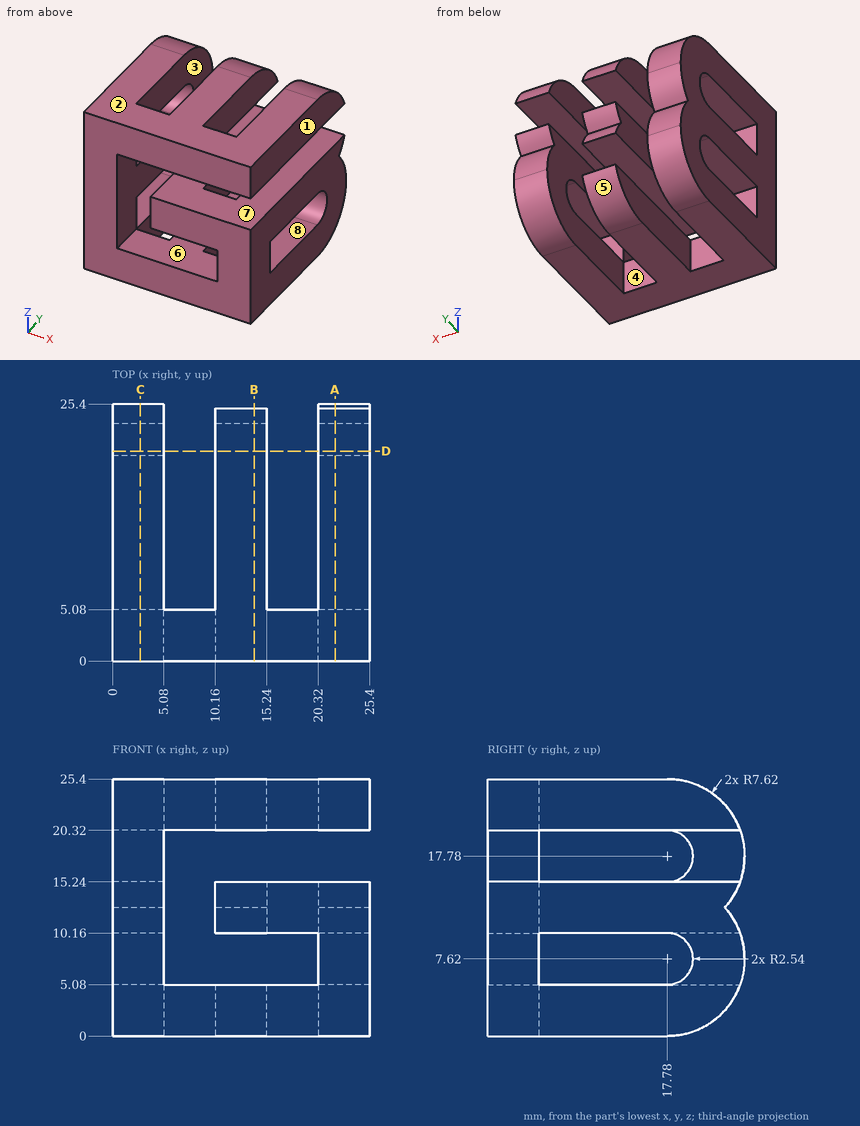
Verification items for this drawing (mm, ordinates from the low corner). A direction names the side the tool comes from. Round coordinates to 2 decimals unless told otherwise and drop trailing zeros. Write each loop counter-clockwise with the first axis right and the second up, starting at its lowest first coordinate (ties: lowest second). Pieces come first, ordered by that corner, then holes. Notation, with made-up numbers: (23.25, 17) - (45.25, 17) arc R14 cw to (45.25, 25) - close; hole circle Ø9 at (61.25, 49). An arc over 180 degrees is marked (long way). One line per item, written item: value.
1. Depth check by flat-ended pin: pin 1 Ø6 at (x, y) = (14.5, 18.5) entering from -Z; pin 2 Ø1.5 at (x, z) = (18, 13.5) entering from +Y; pin 3 Ø8 at (x, y) = (22.5, 22) entering from +Z; pin 4 Ø5 at (x, y) = (9.5, 21.5) entering from -Z. Enter the tip coordinate at first touch or a pass-through.
The answers:
pin 1: stops at z = 0
pin 2: stops at y = 5.08
pin 3: stops at z = 25.4
pin 4: stops at z = 0.11
2. Cross-section at A-A on x = 22. Record the boundary of the cut face in (y, z), and give its area (3 significant figures).
The answers:
outline: (0, 0) - (17.78, 0) arc R7.62 ccw to (23.46, 12.7) arc R7.62 ccw to (24.96, 15.24) - (0, 15.24) - close; (0, 20.32) - (24.96, 20.32) arc R7.62 ccw to (17.78, 25.4) - (0, 25.4) - close; hole (5.08, 5.08) - (17.78, 5.08) arc R2.54 ccw to (17.78, 10.16) - (5.08, 10.16) - close
area: 411 mm^2
3. Cross-section at B-B on x = 14. Record the boundary of the cut face in (y, z).
The answers:
outline: (0, 0) - (17.78, 0) arc R7.62 ccw to (24.96, 5.08) - (0, 5.08) - close; (0, 10.16) - (24.96, 10.16) arc R7.62 ccw to (23.46, 12.7) arc R7.62 ccw to (24.96, 15.24) - (0, 15.24) - close; (0, 20.32) - (24.96, 20.32) arc R7.62 ccw to (17.78, 25.4) - (0, 25.4) - close
4. Mould release check, pull along X, two halves, no side actions. Record for the marked faces 1, 2 and 3: released by +X, released by -X, zero draft, split by the parting line, or undercut.
The answers:
face 1: released by +X
face 2: zero draft
face 3: undercut
5. Cross-section at D-D on y = 20.75. Record the boundary of the cut face in (x, z).
The answers:
outline: (0, 0.6) - (5.08, 0.6) - (5.08, 24.8) - (0, 24.8) - close; (10.16, 0.6) - (15.24, 0.6) - (15.24, 5.08) - (10.16, 5.08) - close; (10.16, 10.16) - (15.24, 10.16) - (15.24, 15.24) - (10.16, 15.24) - close; (10.16, 20.32) - (15.24, 20.32) - (15.24, 24.8) - (10.16, 24.8) - close; (20.32, 0.6) - (25.4, 0.6) - (25.4, 15.24) - (20.32, 15.24) - close; (20.32, 20.32) - (25.4, 20.32) - (25.4, 24.8) - (20.32, 24.8) - close
6. Set-up check for the marked faces 4, 5, 6, 7 and 8: record each of +Z, -Z, +X, -X, +Y, -Y from which the full face is reachable in a straight line by a thin tool's end or side.
The answers:
face 4: +Z, -Z, +Y
face 5: -Z, +X, -X, +Y
face 6: +Y, -Y
face 7: +X, +Y, -Y
face 8: +X, -X
7. Cross-section at C-C on x = 2.75. Record the boundary of the cut face in (y, z).
The answers:
outline: (0, 0) - (17.78, 0) arc R7.62 ccw to (23.46, 12.7) arc R7.62 ccw to (17.78, 25.4) - (0, 25.4) - close; hole (5.08, 5.08) - (17.78, 5.08) arc R2.54 ccw to (17.78, 10.16) - (5.08, 10.16) - close; hole (5.08, 15.24) - (17.78, 15.24) arc R2.54 ccw to (17.78, 20.32) - (5.08, 20.32) - close
8. Scan lines: L1, parallel to X at y = 22.25, z = 23; L2, parallel to X at y = 4.5, z = 9. Record each from-to range of solid material in increasing order.
The answers:
L1: x = 0 to 5.08, 10.16 to 15.24, 20.32 to 25.4
L2: x = 0 to 5.08, 20.32 to 25.4
